Drawing for the job (mm, zero at the part's lowest x, y, z). A direction names the side the tool comes from. Round coordinates to 2 decimals unless told otherwise and drop trailing zeros. Write each loop counter-clockwise with the first axis right and the second up, starting at its lowest first coordinate (ties: lowest second). Pieces come first, ordered by that corner, then holes.
Item 1: Band-saw the part on C-C, the plane z = 35.5. Write the cut outline in (x, y).
Item 2: Band-saw the part on D-D, the plane z = 17.5. Write the cut outline in (x, y), then the cut area to 3 significant figures.
Item 3: 3-axis set-ups, long thin cutter, end or side, ignore diameter. For the marked faces 4, 5 and 6: which of +Z, -Z, +X, -X, +Y, -Y reach the whole face in a straight line?
Item 4: Band-saw the part on B-B, the plane x = 45. Write the cut outline in (y, z).
Item 5: Drop flat-ended pins along their axis: pin 1 Ø8 at (y, z) = (20, 12.5) entering from +X; pin 2 Ø8.5 at (y, z) = (15.5, 36) entering from -X; pin 3 Ø4 at (y, z) = (18, 26.5) entering from -X (1 decimal). Give the stop position or say it passes through.
Item 6: Mould opens along X. For the marked faces 1, 2 and 3 say: +X half, -X half, draft (parallel to the pull), parting line (faces both ways), or undercut.
Item 7: Band-saw the part on A-A, the plane y = 18. Write the cut outline in (x, z).
Item 8: Wall check: probe 1 along X at (y, z) = (17, 40); probe 2 along X at (y, z) = (29, 34); probe 3 along Z at (x, y) = (29, 30.5). Give the ranges that are in metal, low to high.
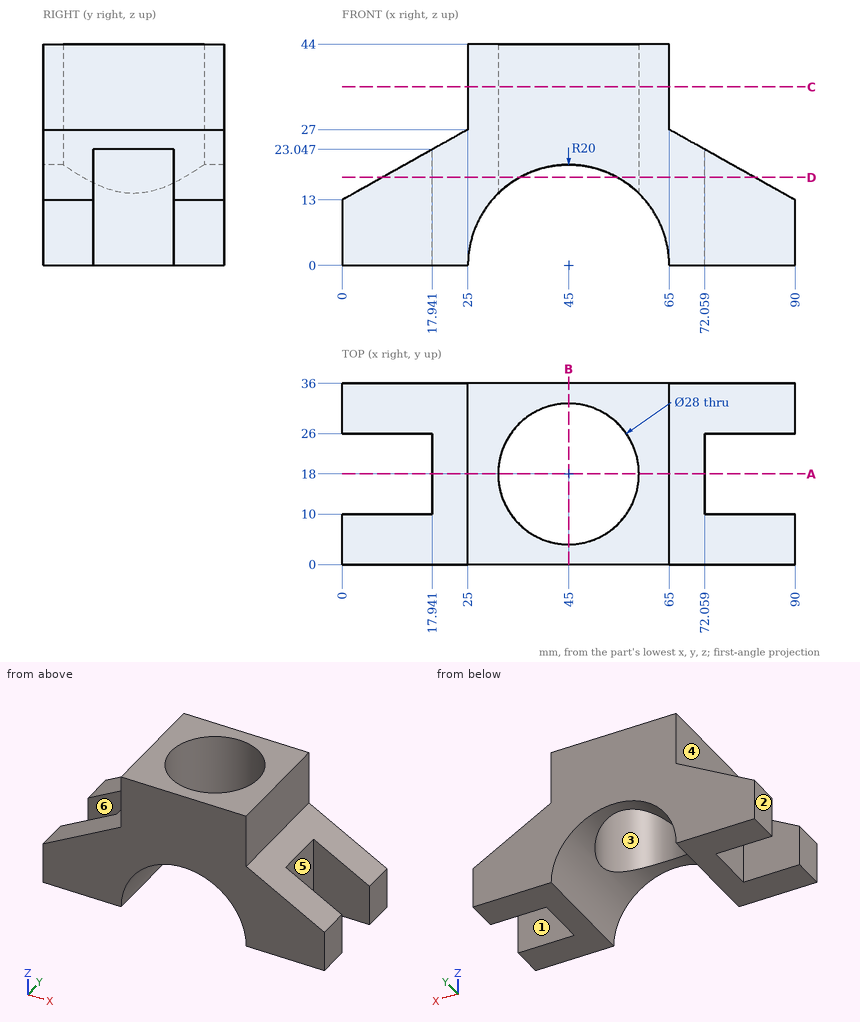
Results:
1. outline: (25, 0) - (65, 0) - (65, 36) - (25, 36) - close; hole circle Ø28 at (45, 18)
2. outline: (8.04, 0) - (35.32, 0) - (35.32, 7.89) arc R14 cw to (35.32, 28.11) - (35.32, 36) - (8.04, 36) - (8.04, 26) - (17.94, 26) - (17.94, 10) - (8.04, 10) - close; (54.68, 0) - (81.96, 0) - (81.96, 10) - (72.06, 10) - (72.06, 26) - (81.96, 26) - (81.96, 36) - (54.68, 36) - (54.68, 28.11) arc R14 cw to (54.68, 7.89) - close
2. area: 1,530 mm2
3. face 4: +Z, -X, +Y, -Y
3. face 5: +Z, -Z, +X
3. face 6: +Z, -Z, -X
4. outline: (0, 20) - (4, 20) - (4, 44) - (0, 44) - close; (32, 20) - (36, 20) - (36, 44) - (32, 44) - close
5. pin 1: stops at x = 72.06
5. pin 2: stops at x = 25
5. pin 3: stops at x = 20.5
6. face 1: draft
6. face 2: -X half
6. face 3: undercut
7. outline: (17.94, 0) - (25, 0) arc R20 cw to (31, 14.28) - (31, 44) - (25, 44) - (25, 27) - (17.94, 23.05) - close; (59, 14.28) arc R20 cw to (65, 0) - (72.06, 0) - (72.06, 23.05) - (65, 27) - (65, 44) - (59, 44) - close
8. probe 1: x = 25 to 31.04, 58.96 to 65
8. probe 2: x = 25 to 36.34, 53.66 to 65
8. probe 3: z = 12 to 44
